```python
from build123d import *

# Parameters (mm, degrees)
F1_DEPTH = 12.7
F2_R     = 5.08
F3_R     = 31.75
F4_R     = 12.7
F5_DEPTH = 25.4


with BuildPart() as f1:
    # F0 (on Front) → F1 (new body, symmetric)
    with BuildSketch(Plane.XZ):
        Polygon((38.1, 38.1), (-38.1, 38.1), (-38.1, -12.7), (0, -12.7), (38.1, -12.7), align=None)
        Polygon((-38.1, -12.7), (-63.5, -12.7), (-63.5, -38.1), (63.5, -38.1), (63.5, -12.7), (38.1, -12.7), (0, -12.7), align=None)
    extrude(amount=F1_DEPTH, both=True)

    # F2
    f2_edges = [f1.edges().sort_by_distance(p)[0] for p in [
        (-63.5, 0, -12.7),
        (63.5, 0, -12.7),
        (-38.1, 0, -12.7),
        (38.1, 0, -12.7),
    ]]
    fillet(f2_edges, radius=F2_R)

    # F3
    f3_edges = [f1.edges().sort_by_distance(p)[0] for p in [
        (-38.1, 0, 38.1),
        (38.1, 0, 38.1),
    ]]
    fillet(f3_edges, radius=F3_R)

    # F4 (on Front) → F5 (cut, symmetric)
    with BuildSketch(Plane.XZ):
        with Locations((0, 9.525)):
            Circle(F4_R)
    extrude(amount=F5_DEPTH, both=True, mode=Mode.SUBTRACT)


solid = f1.part
```
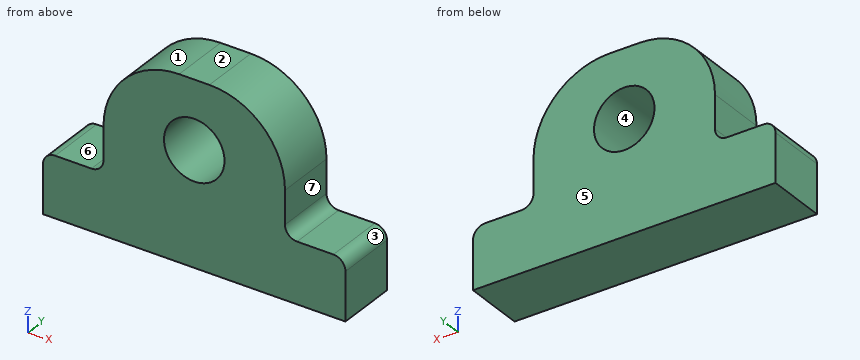
Input: part model. Units: mm. Frame: model coordinates. Face numbers are marked on the shaded views. A direction names the side the tool comes from. Give positions to 0.01 mm unless a question says otherwise; leave off trailing zeros. Order: outer loops, then holes, each group sorted by start corner. A loop starts at its lowest first (then second) coordinate and runs counter-clockwise, first axis right, second up.
1. Reachability of the marked faces 5, 6 and 7 from +Z, -Z, +X, -X, +Y, -Y: full face, straight path, thin tool, end or side. Return the list, or none.
Derived:
face 5: +Z, -Z, +X, -X, +Y
face 6: +Z, -X, +Y, -Y
face 7: +Z, +X, +Y, -Y
2. Section A-A on x = 0. Return the cut outline in (y, z) (3 decimals), and give its area (3 significant figures).
Derived:
outline: (-12.7, -38.1) - (12.7, -38.1) - (12.7, -3.175) - (-12.7, -3.175) - close; (-12.7, 22.225) - (12.7, 22.225) - (12.7, 38.1) - (-12.7, 38.1) - close
area: 1,290 mm2
3. Mould query, pull axis X, two halves, no side actions, for the marked faces 1, 2, 3 and 4. Classes: released by +X, released by -X, zero draft, split by the parting line, or undercut.
Derived:
face 1: released by -X
face 2: zero draft
face 3: released by +X
face 4: undercut
4. Section C-C on x = -54. Return the cut outline in (y, z).
Derived:
outline: (-12.7, -38.1) - (12.7, -38.1) - (12.7, -12.7) - (-12.7, -12.7) - close
5. Material intervals for L1, parallel to Z at x = 0, y = -6.25 (3 decimals); L2, parallel to X at y = -3.5, z = 5; L3, parallel to X at y = -5, z = -5, sorted ascending.
Derived:
L1: z = -38.1 to -3.175, 22.225 to 38.1
L2: x = -38.1 to -11.87, 11.87 to 38.1
L3: x = -38.1 to 38.1
6. Section D-D on x = -15.5. Return the cut outline in (y, z).
Derived:
outline: (-12.7, -38.1) - (12.7, -38.1) - (12.7, 36.75) - (-12.7, 36.75) - close
7. Section B-B on y = -10.5. Return the cut outline in (x, z) (3 decimals).
Derived:
outline: (-63.5, -38.1) - (63.5, -38.1) - (63.5, -17.78) arc R5.08 ccw to (58.42, -12.7) - (43.18, -12.7) arc R5.08 cw to (38.1, -7.62) - (38.1, 6.35) arc R31.75 ccw to (6.35, 38.1) - (-6.35, 38.1) arc R31.75 ccw to (-38.1, 6.35) - (-38.1, -7.62) arc R5.08 cw to (-43.18, -12.7) - (-58.42, -12.7) arc R5.08 ccw to (-63.5, -17.78) - close; hole circle Ø25.4 at (0, 9.525)
8. Pin query (flat end, axial travel): pin 1 (1.5 mm diameter, centred on x = -32, y = -8.5, fed in from +Z); pin 2 (5 mm diameter, centred on x = -27, y = 8.5, fed in from +Z); pin 3 (12 mm diameter, centred on x = -52, y = 5.5, fed in from +Z); pin 4 (23 mm diameter, centred on x = 0, z = 9.525, fed in from -Y). Return the tip coordinate at first contact, or that it passes through.
Derived:
pin 1: stops at z = 26.05
pin 2: stops at z = 32.4
pin 3: stops at z = -12.7
pin 4: passes through
